```python
from build123d import *

# Parameters (mm, degrees)
BOSS_EXTRUDE1_DEPTH = 2
SKETCH2_W           = 2
SKETCH2_H           = 15
BOSS_EXTRUDE2_DEPTH = 10
FILLET1_R           = 1
FILLET2_R           = 1


with BuildPart() as part:
    # Sketch1 → Boss-Extrude1 (new body)
    with BuildSketch(Plane(origin=(0, 0, 0), x_dir=(1, 0, 0), z_dir=(0, 1, 0))):
        with BuildLine():
            Line((33, 7.5), (21.5, 7.5))
            ThreePointArc((21.5, 7.5), (20, 6), (18.5, 7.5))
            Line((18.5, 7.5), (11.5, 7.5))
            ThreePointArc((11.5, 7.5), (10, 6), (8.5, 7.5))
            Line((8.5, 7.5), (0, 7.5))
            Line((0, 7.5), (0, 0))
            Line((0, 0), (33, 0))
            Line((33, 0), (33, 7.5))
        make_face()
        with BuildLine():
            ThreePointArc((18.5, 7.5), (20, 9), (21.5, 7.5))
            Line((21.5, 7.5), (33, 7.5))
            Line((33, 7.5), (33, 15))
            Line((33, 15), (0, 15))
            Line((0, 15), (0, 7.5))
            Line((0, 7.5), (8.5, 7.5))
            ThreePointArc((8.5, 7.5), (10, 9), (11.5, 7.5))
            Line((11.5, 7.5), (18.5, 7.5))
        make_face()
    extrude(amount=BOSS_EXTRUDE1_DEPTH)

    # Sketch2 → Boss-Extrude2 (add)
    with BuildSketch(Plane(origin=(0, 2, 0), x_dir=(1, 0, 0), z_dir=(0, 1, 0))):
        with Locations((32, 7.5)):
            Rectangle(SKETCH2_W, SKETCH2_H)
    extrude(amount=BOSS_EXTRUDE2_DEPTH)

    # Fillet1
    fillet1_edges = [part.edges().sort_by_distance(p)[0] for p in [
        (0, 1, 0),
        (0, 1, -15),
        (31, 2, -7.5),
        (32, 12, -15),
        (32, 12, 0),
    ]]
    fillet(fillet1_edges, radius=FILLET1_R)

    # Fillet2
    fillet2_edges = [part.edges().sort_by_distance(p)[0] for p in [
        (33, 0, -7.5),
    ]]
    fillet(fillet2_edges, radius=FILLET2_R)


solid = part.part
```
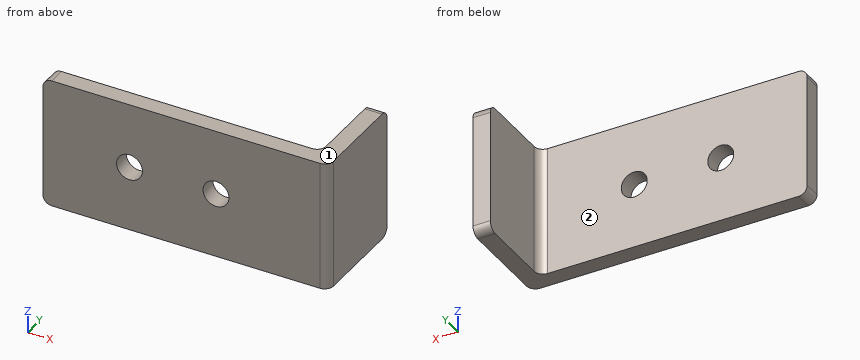
Geometry check sheet. Reference: the model listing, model coordinates, mm. Face numbers are marked on the shaded views. A direction names the side the tool comes from. Give positions to 0.01 mm unless a question says otherwise; leave off trailing zeros. Order: outer loops, then holes, each group sorted by start corner. A loop starts at its lowest first (then second) coordinate and runs counter-clockwise, first axis right, second up.
1. Thickness scan on L1, parallel to X at y = 1.15, z = -7.5; L2, parallel to Z at x = 20, y = 1.6; L3, parallel to X at y = 0.4, z = -7.5. Record the ranges inside material, lowest first.
2. Section check A-A, the plane x = 20. Enter the section's corners in (y, z), and give its area (3 significant figures).
3. Access from +Z, -Z, +X, -X, +Y, -Y to the whole of each face (thin tool, end or side, straight path). Record for the marked faces 1 and 2.
4. Gauge pin test, flat ends, axial feed: pin 1 Ø4 at (x, z) = (10, -7.5) entering from +Y; pin 2 Ø2.5 at (y, z) = (8.5, -11) entering from -X. Record the tip position at first contact, or that the pin passes through.
5. Section check B-B, the plane z = -7.5. Enter the section's corners in (x, y), and give its area (3 significant figures).
6. Section check D-D, the plane y = 5.5. Enter the section's corners in (x, z).
7. Section check C-C, the plane z = -1.5. Enter the section's corners in (x, y), and give its area (3 significant figures).
Values follow:
1. L1: x = 0 to 8.5, 11.5 to 18.5, 21.5 to 33
1. L2: z = -15 to -9, -6 to 0
1. L3: x = 0 to 8.5, 11.5 to 18.5, 21.5 to 32.8
2. outline: (0, -15) - (2, -15) - (2, -9) - (0, -9) - close; (0, -6) - (2, -6) - (2, 0) - (0, 0) - close
2. area: 24.0 mm2
3. face 1: +Z, +X, -X, +Y, -Y
3. face 2: +Z, -Z, -X, +Y
4. pin 1: stops at y = 2
4. pin 2: stops at x = 31
5. outline: (0, 0) - (8.5, 0) - (8.5, 2) - (0, 2) - close; (11.5, 0) - (18.5, 0) - (18.5, 2) - (11.5, 2) - close; (21.5, 0) - (32, 0) arc R1 ccw to (33, 1) - (33, 12) - (31, 12) - (31, 3) arc R1 cw to (30, 2) - (21.5, 2) - close
5. area: 74.0 mm2
6. outline: (31, -15) - (33, -15) - (33, 0) - (31, 0) - close
7. outline: (0, 0) - (32, 0) arc R1 ccw to (33, 1) - (33, 12) - (31, 12) - (31, 3) arc R1 cw to (30, 2) - (0, 2) - close
7. area: 86.0 mm2
